from build123d import *

# Parameters (mm, degrees)
SKETCH1_W                                            = 300
SKETCH1_H                                            = 210
BOSS_EXTRUDE1_DEPTH                                  = 10
SKETCH2_W                                            = 280
SKETCH2_H                                            = 190
BOSS_EXTRUDE2_DEPTH                                  = 9.28
F_1_4_20_CLEARANCE_HOLES_REACH                       = 21.28
SKETCH3_R                                            = 3.57
SKETCH4_R                                            = 7.5
CUT_EXTRUDE2_DEPTH                                   = 10
SKETCH5_R                                            = 1.13
F_4_40_THREADED_HOLES_DEPTH                          = 5
SKETCH6_R                                            = 1.13
F_4_40_THREADED_HOLES_2_DEPTH                        = 5
SKETCH7_R                                            = 1.13
F_4_40_THREADED_HOLES_3_DEPTH                        = 5
SKETCH8_R                                            = 1.13
F_4_40_THREADED_HOLES_4_DEPTH                        = 5
SKETCH11_W                                           = 54
SKETCH11_H                                           = 51
TEC_DEPTH                                            = 1
FILLET1_R                                            = 2
OPTICAL_TABLE_CBORE_FOR_1_4_BINDING_HEAD_D           = 7.14248
OPTICAL_TABLE_CBORE_FOR_1_4_BINDING_HEAD_DEPTH       = 19.28
OPTICAL_TABLE_CBORE_FOR_1_4_BINDING_HEAD_CBORE_D     = 14.2875
OPTICAL_TABLE_CBORE_FOR_1_4_BINDING_HEAD_CBORE_DEPTH = 4.191


with BuildPart() as part:
    # Sketch1 → Boss-Extrude1 (new body)
    with BuildSketch(Plane(origin=(0, 0, 0), x_dir=(1, 0, 0), z_dir=(0, 1, 0))):
        with Locations((-22.864321608, -2.487437186)):
            Rectangle(SKETCH1_W, SKETCH1_H)
    extrude(amount=BOSS_EXTRUDE1_DEPTH)

    # Sketch2 → Boss-Extrude2 (add)
    with BuildSketch(Plane(origin=(0, 10, 0), x_dir=(1, 0, 0), z_dir=(0, 1, 0))):
        with Locations((-22.864321608, -2.487437186)):
            Rectangle(SKETCH2_W, SKETCH2_H)
    extrude(amount=BOSS_EXTRUDE2_DEPTH)

    # Sketch3 → 1/4-20 clearance holes (cut, up to next)
    with BuildSketch(Plane(origin=(0, 19.28, 0), x_dir=(1, 0, 0), z_dir=(0, 1, 0)), mode=Mode.PRIVATE) as f_1_4_20_clearance_holes_sk1:
        with Locations((-122.864321608, 65.012562814)):
            Circle(SKETCH3_R)
    f_1_4_20_clearance_holes_tool1 = extrude(f_1_4_20_clearance_holes_sk1.sketch, amount=-F_1_4_20_CLEARANCE_HOLES_REACH, mode=Mode.PRIVATE) & part.part
    add(f_1_4_20_clearance_holes_tool1.solids().sort_by_distance((-122.864322, 19.28, -65.012563))[0], mode=Mode.SUBTRACT)
    # Sketch3 → 1/4-20 clearance holes (cut, up to next)
    with BuildSketch(Plane(origin=(0, 19.28, 0), x_dir=(1, 0, 0), z_dir=(0, 1, 0)), mode=Mode.PRIVATE) as f_1_4_20_clearance_holes_sk2:
        with Locations((-39.114321608, 65.012562814)):
            Circle(SKETCH3_R)
    f_1_4_20_clearance_holes_tool2 = extrude(f_1_4_20_clearance_holes_sk2.sketch, amount=-F_1_4_20_CLEARANCE_HOLES_REACH, mode=Mode.PRIVATE) & part.part
    add(f_1_4_20_clearance_holes_tool2.solids().sort_by_distance((-39.114322, 19.28, -65.012563))[0], mode=Mode.SUBTRACT)
    # Sketch3 → 1/4-20 clearance holes (cut, up to next)
    with BuildSketch(Plane(origin=(0, 19.28, 0), x_dir=(1, 0, 0), z_dir=(0, 1, 0)), mode=Mode.PRIVATE) as f_1_4_20_clearance_holes_sk3:
        with Locations((44.635678392, 65.012562814)):
            Circle(SKETCH3_R)
    f_1_4_20_clearance_holes_tool3 = extrude(f_1_4_20_clearance_holes_sk3.sketch, amount=-F_1_4_20_CLEARANCE_HOLES_REACH, mode=Mode.PRIVATE) & part.part
    add(f_1_4_20_clearance_holes_tool3.solids().sort_by_distance((44.635678, 19.28, -65.012563))[0], mode=Mode.SUBTRACT)
    # Sketch3 → 1/4-20 clearance holes (cut, up to next)
    with BuildSketch(Plane(origin=(0, 19.28, 0), x_dir=(1, 0, 0), z_dir=(0, 1, 0)), mode=Mode.PRIVATE) as f_1_4_20_clearance_holes_sk4:
        with Locations((44.635678392, -69.987437186)):
            Circle(SKETCH3_R)
    f_1_4_20_clearance_holes_tool4 = extrude(f_1_4_20_clearance_holes_sk4.sketch, amount=-F_1_4_20_CLEARANCE_HOLES_REACH, mode=Mode.PRIVATE) & part.part
    add(f_1_4_20_clearance_holes_tool4.solids().sort_by_distance((44.635678, 19.28, 69.987437))[0], mode=Mode.SUBTRACT)
    # Sketch3 → 1/4-20 clearance holes (cut, up to next)
    with BuildSketch(Plane(origin=(0, 19.28, 0), x_dir=(1, 0, 0), z_dir=(0, 1, 0)), mode=Mode.PRIVATE) as f_1_4_20_clearance_holes_sk5:
        with Locations((-39.114321608, -69.987437186)):
            Circle(SKETCH3_R)
    f_1_4_20_clearance_holes_tool5 = extrude(f_1_4_20_clearance_holes_sk5.sketch, amount=-F_1_4_20_CLEARANCE_HOLES_REACH, mode=Mode.PRIVATE) & part.part
    add(f_1_4_20_clearance_holes_tool5.solids().sort_by_distance((-39.114322, 19.28, 69.987437))[0], mode=Mode.SUBTRACT)
    # Sketch3 → 1/4-20 clearance holes (cut, up to next)
    with BuildSketch(Plane(origin=(0, 19.28, 0), x_dir=(1, 0, 0), z_dir=(0, 1, 0)), mode=Mode.PRIVATE) as f_1_4_20_clearance_holes_sk6:
        with Locations((-122.864321608, -69.987437186)):
            Circle(SKETCH3_R)
    f_1_4_20_clearance_holes_tool6 = extrude(f_1_4_20_clearance_holes_sk6.sketch, amount=-F_1_4_20_CLEARANCE_HOLES_REACH, mode=Mode.PRIVATE) & part.part
    add(f_1_4_20_clearance_holes_tool6.solids().sort_by_distance((-122.864322, 19.28, 69.987437))[0], mode=Mode.SUBTRACT)

    # Sketch4 → Cut-Extrude2 (cut)
    with BuildSketch(Plane.XZ):
        with Locations((-122.864321608, 69.987437186)):
            Circle(SKETCH4_R)
        with Locations((-39.114321608, 69.987437186)):
            Circle(SKETCH4_R)
        with Locations((44.635678392, 69.987437186)):
            Circle(SKETCH4_R)
        with Locations((44.635678392, -65.012562814)):
            Circle(SKETCH4_R)
        with Locations((-39.114321608, -65.012562814)):
            Circle(SKETCH4_R)
        with Locations((-122.864321608, -65.012562814)):
            Circle(SKETCH4_R)
    extrude(amount=-CUT_EXTRUDE2_DEPTH, mode=Mode.SUBTRACT)

    # Sketch5 → 4-40 threaded holes (cut)
    with BuildSketch(Plane.XY.offset(97.487437186)):
        with Locations((-147.864321608, 14.64)):
            Circle(SKETCH5_R)
        with Locations((-22.864321608, 14.64)):
            Circle(SKETCH5_R)
        with Locations((102.135678392, 14.64)):
            Circle(SKETCH5_R)
    extrude(amount=-F_4_40_THREADED_HOLES_DEPTH, mode=Mode.SUBTRACT)

    # Sketch6 → 4-40 threaded holes 2 (cut)
    with BuildSketch(Plane(origin=(0, 0, -92.512562814), x_dir=(-1, 0, 0), z_dir=(0, 0, -1))):
        with Locations((-102.135678392, 14.64)):
            Circle(SKETCH6_R)
        with Locations((22.864321608, 14.64)):
            Circle(SKETCH6_R)
        with Locations((147.864321608, 14.64)):
            Circle(SKETCH6_R)
    extrude(amount=-F_4_40_THREADED_HOLES_2_DEPTH, mode=Mode.SUBTRACT)

    # Sketch7 → 4-40 threaded holes 3 (cut)
    with BuildSketch(Plane.ZY.offset(162.864321608)):
        with Locations((-62.512562814, 14.64)):
            Circle(SKETCH7_R)
        with Locations((2.487437186, 14.64)):
            Circle(SKETCH7_R)
        with Locations((67.487437186, 14.64)):
            Circle(SKETCH7_R)
    extrude(amount=-F_4_40_THREADED_HOLES_3_DEPTH, mode=Mode.SUBTRACT)

    # Sketch8 → 4-40 threaded holes 4 (cut)
    with BuildSketch(Plane(origin=(117.135678392, 0, 0), x_dir=(0, 0, -1), z_dir=(1, 0, 0))):
        with Locations((-67.487437186, 14.64)):
            Circle(SKETCH8_R)
        with Locations((-2.487437186, 14.64)):
            Circle(SKETCH8_R)
        with Locations((62.512562814, 14.64)):
            Circle(SKETCH8_R)
    extrude(amount=-F_4_40_THREADED_HOLES_4_DEPTH, mode=Mode.SUBTRACT)

    # Sketch11 → TEC (cut)
    with BuildSketch(Plane(origin=(0, 19.28, 0), x_dir=(1, 0, 0), z_dir=(0, 1, 0))):
        with Locations((-17.563304852, 24.512562814)):
            Rectangle(SKETCH11_W, SKETCH11_H)
        with Locations((-80.864321608, -44.487437186)):
            Rectangle(SKETCH11_W, SKETCH11_H)
        with Locations((2.635678392, -44.487437186)):
            Rectangle(SKETCH11_W, SKETCH11_H)
    extrude(amount=-TEC_DEPTH, mode=Mode.SUBTRACT)

    # Fillet1
    fillet1_edges = [part.edges().sort_by_distance(p)[0] for p in [
        (9.436695148, 18.78, -50.012562814),
        (9.436695148, 18.78, 0.987437186),
        (-44.563304852, 18.78, 0.987437186),
        (-44.563304852, 18.78, -50.012562814),
        (-53.864321608, 18.78, 69.987437186),
        (-107.864321608, 18.78, 69.987437186),
        (-107.864321608, 18.78, 18.987437186),
        (-53.864321608, 18.78, 18.987437186),
        (29.635678392, 18.78, 69.987437186),
        (-24.364321608, 18.78, 69.987437186),
        (-24.364321608, 18.78, 18.987437186),
        (29.635678392, 18.78, 18.987437186),
    ]]
    fillet(fillet1_edges, radius=FILLET1_R)

    # optical table CBORE for 1/4 Binding Head Machine Screw1
    with Locations(Plane(origin=(0, 19.28, 0), x_dir=(1, 0, 0), z_dir=(0, 1, 0))):
        with Locations((-147.864321608, 61.012562814), (-147.864321608, -65.987437186), (80.735678392, -65.987437186), (80.735678392, 61.012562814)):
            CounterBoreHole(OPTICAL_TABLE_CBORE_FOR_1_4_BINDING_HEAD_D / 2, OPTICAL_TABLE_CBORE_FOR_1_4_BINDING_HEAD_CBORE_D / 2, OPTICAL_TABLE_CBORE_FOR_1_4_BINDING_HEAD_CBORE_DEPTH, depth=OPTICAL_TABLE_CBORE_FOR_1_4_BINDING_HEAD_DEPTH)


solid = part.part
The model under review builds one solid part; all positions refer to its coordinate system, in mm. A direction names the side the tool comes from. Round coordinates to 2 decimals unless told otherwise and drop trailing zeros. Loops run counter-clockwise (first coordinate to the right, second up) from the corner with the lowest first, then second, coordinate; pieces in that order, holes last. Notation, with made-up numbers: M 9,-5 L 47,-5 A28 ccw 47,28 Z; hole C -4,76 d11. An arc over 180 degrees is marked long. Answer as CSV lines item,"result".
1. Draft analysis for pull direction X (two halves, no side actions). For faces 5 (the face through (-35, 10, 103)), 6 (the face through (-145, 15.089, 69)), 7 (the face through (127.136, 5, 4)), state which applies: pulls with the +X half, pulls with the -X half, needs draft (parallel to the pull), parting line crosses it, or undercut.
Outcome:
face 5,"needs draft"
face 6,"undercut"
face 7,"pulls with the +X half"
2. We need section A-A (x = 2.5). Give the boundary of the cut face in (y, z), plus the area to 3 significant figures.
Outcome:
outline,"M 0,-102.51 L 10,-102.51 L 10,-92.51 L 19.28,-92.51 L 19.28,-50.01 L 18.28,-50.01 L 18.28,0.99 L 19.28,0.99 L 19.28,18.99 L 18.28,18.99 L 18.28,69.99 L 19.28,69.99 L 19.28,97.49 L 10,97.49 L 10,107.49 L 0,107.49 Z"
area,"3,760 mm2"
3. Insertion check: pin 1 Ø2.5 at (y, z) = (14.64, -62.51) entering from +X; pin 2 Ø3 at (x, z) = (-105, 44) entering from +Y; pin 3 Ø3 at (x, y) = (-138.5, 15.5) entering from +Z; pin 4 Ø4.5 at (x, z) = (-39.5, -64.5) entering from -Y. Each pin has a flat end and moves straight along its axis. Give the tip position at first contact, or say it passes through.
Outcome:
pin 1,"stops at x = 117.14"
pin 2,"stops at y = 18.28"
pin 3,"stops at z = 97.49"
pin 4,"passes through"
4. We need section C-C (x = -60). Give the boundary of the cut face in (y, z).
Outcome:
outline,"M 0,-102.51 L 10,-102.51 L 10,-92.51 L 19.28,-92.51 L 19.28,18.99 L 18.28,18.99 L 18.28,69.99 L 19.28,69.99 L 19.28,97.49 L 10,97.49 L 10,107.49 L 0,107.49 Z"
5. For faces 1 (the face through (-25, 15, -92.513)), 2 (the face through (-40.091, 4.93, -57.576)), 3 (the face through (-162.864, 15, 4)), 4 (the face through (84.576, 17.214, 59.964)), list the 3-axis set-ups (+Z, -Z, +X, -X, +Y, -Y) from which the entire face can be reached by the end or side of a thin tool; tool diameter is ignored.
Outcome:
face 1,"-Z, +X, -X, +Y"
face 2,"-Y"
face 3,"+Z, -Z, -X, +Y"
face 4,"+Y"
6. We need section B-B (z = 31). Give the boundary of the cut face in (x, y), plus the area to 3 significant figures.
Outcome:
outline,"M -172.86,0 L 127.14,0 L 127.14,10 L 117.14,10 L 117.14,19.28 L 29.64,19.28 L 29.64,18.28 L -24.36,18.28 L -24.36,19.28 L -53.86,19.28 L -53.86,18.28 L -107.86,18.28 L -107.86,19.28 L -162.86,19.28 L -162.86,10 L -172.86,10 Z"
area,"5,490 mm2"
7. To check wall thickness, follow L1, parallel to X at y = 7, z = 68; L2, parallel to Z at x = 16, y = 13.5; L3, parallel to X at y = 16, z = 92. State the ranges of each line that lie inside material, in increasing order. Write a range as [from, to].
Outcome:
L1,"x = [-172.86, -150.81], [-144.91, -130.1], [-115.63, -46.35], [-31.88, 37.4], [51.87, 77.79], [83.69, 127.14]"
L2,"z = [-92.51, 97.49]"
L3,"x = [-162.86, 117.14]"
